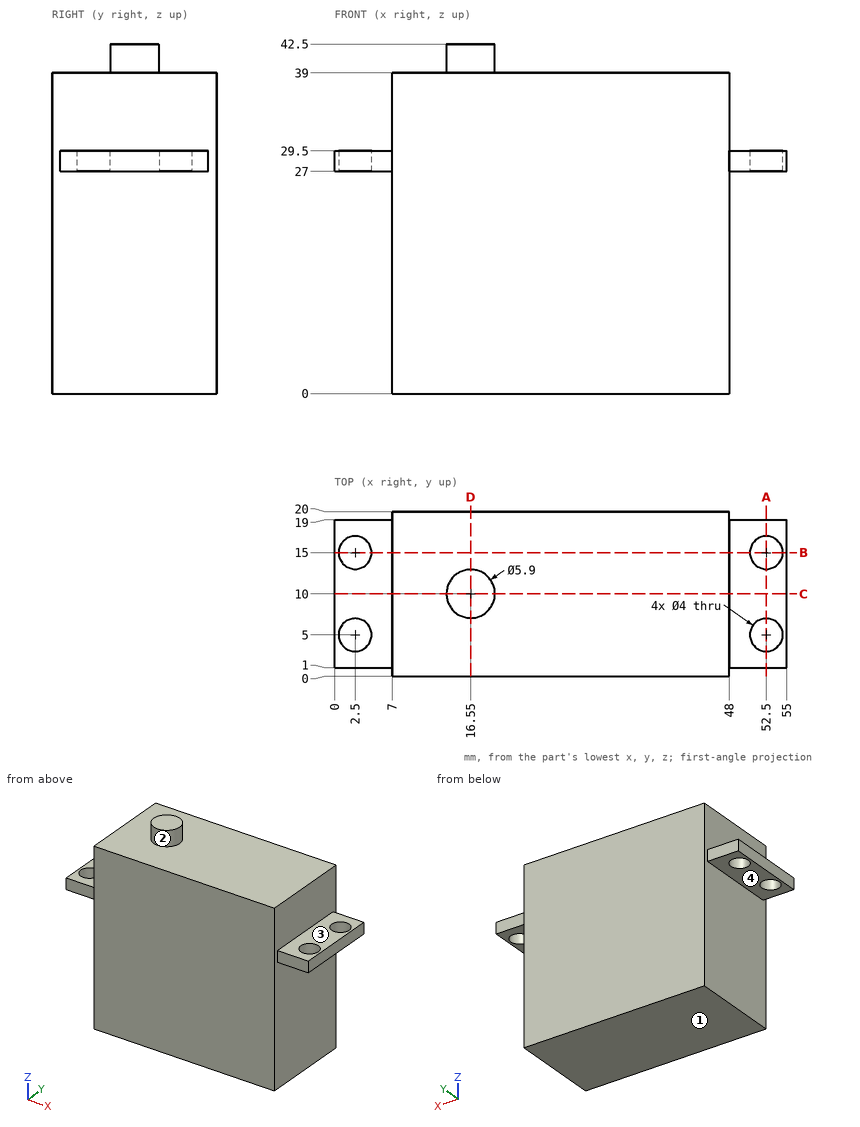
Design review of the part shown in the three views and the two pictorial views. Dimensions are in mm from the part's minimum x, y and z. A direction names the side the tool comes from. Give positions to 0.01 mm unless a question says otherwise; leave off trailing zeros. Write each loop counter-clockwise with the first axis right and the second up, starting at its lowest first coordinate (ties: lowest second). Pieces come first, ordered by that corner, then holes.
(1) Wall thickness on line 1 along Y through (x, z) = (2.5, 28.2); line 2 along Z through (x, y) = (31, 5.25); line 3 along Y through (x, z) = (52, 28): over which ranges is each line inside the solid? List them lowest first.
Checked values:
line 1: y = 1 to 3, 7 to 13, 17 to 19
line 2: z = 0 to 39
line 3: y = 1 to 3.06, 6.94 to 13.06, 16.94 to 19
(2) Add section B-B (y = 15). Give the boundary of the cut face in (x, z), and give its area (3 significant figures).
Checked values:
outline: (0, 27) - (0.5, 27) - (0.5, 29.5) - (0, 29.5) - close; (4.5, 27) - (7, 27) - (7, 0) - (48, 0) - (48, 27) - (50.5, 27) - (50.5, 29.5) - (48, 29.5) - (48, 39) - (7, 39) - (7, 29.5) - (4.5, 29.5) - close; (54.5, 27) - (55, 27) - (55, 29.5) - (54.5, 29.5) - close
area: 1,610 mm2
(3) Add section D-D (x = 16.55). Give the boundary of the cut face in (y, z).
Checked values:
outline: (0, 0) - (20, 0) - (20, 39) - (12.95, 39) - (12.95, 42.5) - (7.05, 42.5) - (7.05, 39) - (0, 39) - close
(4) Tool access review of the marked faces 1, 2, 3 and 4: name each direction out of +Z, -Z, +X, -X, +Y, -Y from which nothing blocks a thin tool from reaching the whole face with its end or side.
Checked values:
face 1: -Z, +X, -X, +Y, -Y
face 2: +Z
face 3: +Z, +X, +Y, -Y
face 4: -Z, -X, +Y, -Y
(5) Add section C-C (y = 10). Give the boundary of the cut face in (x, z).
Checked values:
outline: (0, 27) - (7, 27) - (7, 0) - (48, 0) - (48, 27) - (55, 27) - (55, 29.5) - (48, 29.5) - (48, 39) - (19.5, 39) - (19.5, 42.5) - (13.6, 42.5) - (13.6, 39) - (7, 39) - (7, 29.5) - (0, 29.5) - close
(6) Clearance check with flat-ended pins moving along their axes: pin 1 Ø5.5 at (x, y) = (52.5, 12) entering from +Z; pin 2 Ø2 at (y, z) = (8, 10) entering from -X; pin 3 Ø1.2 at (x, z) = (3.5, 28) entering from +Y. State where each tip first meets the part, or that it passes through.
Checked values:
pin 1: stops at z = 29.5
pin 2: stops at x = 7
pin 3: stops at y = 19
(7) Add section A-A (x = 52.5). Give the boundary of the cut face in (y, z), and give its area (3 significant figures).
Checked values:
outline: (1, 27) - (3, 27) - (3, 29.5) - (1, 29.5) - close; (7, 27) - (13, 27) - (13, 29.5) - (7, 29.5) - close; (17, 27) - (19, 27) - (19, 29.5) - (17, 29.5) - close
area: 25.0 mm2
